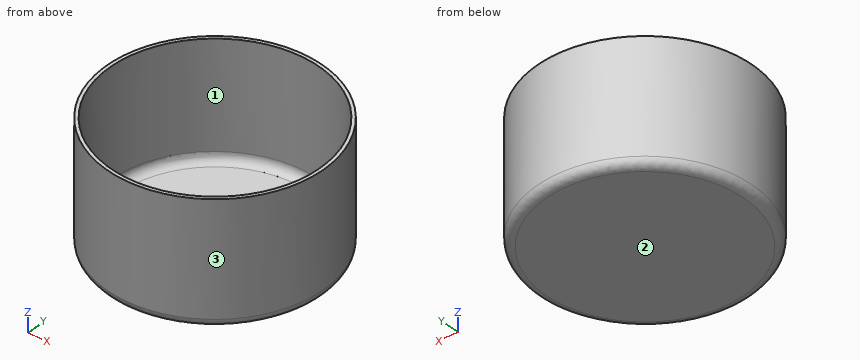
Autodesk Inventor part; units mm, degrees
ref_plane "YZ Plane" through (0, 0, 0) normal (1, 0, 0) x (0, 1, 0)
ref_plane "XZ Plane" through (0, 0, 0) normal (0, 1, 0) x (-1, 0, 0)
ref_plane "XY Plane" through (0, 0, 0) normal (0, 0, 1) x (1, 0, 0)
sketch "Sketch1" plane through (0, 0, 0) normal (0, 0, 1) x (1, 0, 0)
  circle A0 centre (0, 0) radius 20.32
  circle A1 centre (0, 0) radius 19.685
  dimension "d0" = 40.64
  dimension "d1" = 39.37
extrude "Extrusion1" add sketch "Sketch1" along normal blind 21.59
sketch "Sketch2" plane through (0, 0, 0) normal (0, 0, -1) x (-1, 0, 0)
  circle A0 centre (0, 0) radius 20.32
extrude "Extrusion2" add sketch "Sketch2" along normal blind 1.27
fillet "Fillet1" radius 1.5875 2 edges at (20.32, 0, -1.27) (-19.685, 0, 0)
properties part number "PSI Gauge Base 1764"
Geometry: final body of the model. Coordinates: model frame, mm. Face numbers are marked on the shaded views. Round coordinates to 2 decimals unless told otherwise and drop trailing zeros. Write each loop counter-clockwise with the first axis right and the second up, starting at its lowest first coordinate (ties: lowest second). Pieces come first, ordered by that corner, then holes. Notation, with made-up numbers: M -32,71 L -8,71 A31 cw -8,101 Z; hole C 67.5,28.25 d5. An arc over 180 degrees is marked long. Write item = value, one per line.
Item 1: Section query B-B on z = 1. Return loops of the section in (x, y), then the cut area to 3 significant figures.
Findings:
outline = C 0,0 d40.64; hole C 0,0 d39.14
area = 93.7 mm^2
Item 2: Section query A-A on z = 12. Return loops of the section in (x, y) (3 decimals).
Findings:
outline = C 0,0 d40.64; hole C 0,0 d39.37
Item 3: Pull-direction query (Y, two-part tool) for the marked faces 1, 2 and 3; classes: pulls with the +Y half, pulls with the -Y half, needs draft (parallel to the pull), parting line crosses it, or undercut.
Findings:
face_1 = undercut
face_2 = needs draft
face_3 = parting line crosses it
Item 4: Pin query (flat end, axial travel): P1, Ø2, axis at y = -12.5, z = 5.5, coming from the +X side; P2, Ø10, axis at x = -9.5, z = 7.5, coming from the -Y side; P3, Ø3, axis at x = -1.5, z = 7.5, coming from the +Y side; P4, Ø6, axis at x = 11, z = 8, coming from the -Y side. Return the tip coordinate at first contact, or that it passes through.
Findings:
P1 = 16.75
P2 = -19.82
P3 = 20.32
P4 = -18.68
Item 5: Material intervals for line 1 along Y through (x, z) = (0, 6) (3 decimals); line 2 along X through (y, z) = (0.5, 4); line 3 along X through (y, z) = (-10, 11.75), sorted ascending. Write a range as [from, to].
Findings:
line_1 = [-20.32, -19.685], [19.685, 20.32]
line_2 = [-20.31, -19.68], [19.68, 20.31]
line_3 = [-17.69, -16.96], [16.96, 17.69]
